from build123d import *

# Parameters (mm, degrees)
SKETCH1_R                      = 14
BOSS_EXTRUDE1_DEPTH            = 20
CIRPATTERN1_COUNT              = 3
CIRPATTERN1_ANGLE              = 90
M5X0_8_TAPPED_HOLE2_AT_2_COUNT = 2
M5X0_8_TAPPED_HOLE2_AT_2_PITCH = 24
CHAMFER1_SIZE                  = 0.5
FILLET1_R                      = 0.5


with BuildPart() as part:
    # Sketch1 → Boss-Extrude1 (new body, symmetric)
    with BuildSketch(Plane.XY):
        Polygon((-13.25, -19.5), (13.25, -19.5), (26, -6.75), (26, 20), (-26, 20), (-26, -6.75), align=None)
        Circle(SKETCH1_R, mode=Mode.SUBTRACT)
    extrude(amount=BOSS_EXTRUDE1_DEPTH, both=True)

    # Sketch4 → M5x0.8 Tapped Hole1 (revolve, cut)
    with BuildSketch(Plane(origin=(13.435028843, 13.435028843, -20), x_dir=(0, 1, 0), z_dir=(1, 0, 0))):
        Polygon((0, 0), (0, 16.9218073), (2.1, 15.66), (2.1, 0), align=None)
    m5x0_8_tapped_hole1 = revolve(axis=Axis((13.435028843, 13.435028843, -26.35), (0, 0, 1)), mode=Mode.SUBTRACT)

    # CirPattern1: M5x0.8 Tapped Hole1 ×3 about axis
    cirpattern1_axis = Axis((0, 0, 0), (0, 0, -1))
    for i in range(1, CIRPATTERN1_COUNT):
        add(m5x0_8_tapped_hole1.rotate(cirpattern1_axis, i * CIRPATTERN1_ANGLE / (CIRPATTERN1_COUNT - 1)), mode=Mode.SUBTRACT)

    # Mirror1: M5x0.8 Tapped Hole1 across plane
    add(m5x0_8_tapped_hole1.mirror(Plane(origin=(0, 0, 0), x_dir=(0, 0, 1), z_dir=(1, 0, 0))), mode=Mode.SUBTRACT)

    # Mirror1 copy 1 sketch → Mirror1 copy 1 (revolve, cut)
    with BuildSketch(Plane(origin=(-19, 0, -20), x_dir=(-0.707106781, 0.707106781, 0), z_dir=(-0.707106781, -0.707106781, 0))):
        Polygon((0, 0), (0, -16.9218073), (2.1, -15.66), (2.1, 0), align=None)
    revolve(axis=Axis((-19, 0, -26.35), (0, 0, -1)), mode=Mode.SUBTRACT)

    # Mirror1 copy 2 sketch → Mirror1 copy 2 (revolve, cut)
    with BuildSketch(Plane(origin=(-13.435028843, -13.435028843, -20), x_dir=(-1, 0, 0), z_dir=(0, -1, 0))):
        Polygon((0, 0), (0, -16.9218073), (2.1, -15.66), (2.1, 0), align=None)
    revolve(axis=Axis((-13.435028843, -13.435028843, -26.35), (0, 0, -1)), mode=Mode.SUBTRACT)

    # Sketch6 → M5x0.8 Tapped Hole2 (revolve, cut)
    with BuildSketch(Plane(origin=(-20, 20, -12), x_dir=(0, 0, 1), z_dir=(1, 0, 0))):
        Polygon((0, 0), (0, 16.7618073), (2.1, 15.5), (2.1, 0), align=None)
    m5x0_8_tapped_hole2 = revolve(axis=Axis((-20, 26.35, -12), (0, -1, 0)), mode=Mode.SUBTRACT)

    # M5x0.8 Tapped Hole2 at 2: M5x0.8 Tapped Hole2 ×2
    with Locations(*[(0, 0, i * M5X0_8_TAPPED_HOLE2_AT_2_PITCH) for i in range(1, M5X0_8_TAPPED_HOLE2_AT_2_COUNT)]):
        add(m5x0_8_tapped_hole2, mode=Mode.SUBTRACT)

    # Mirror2: M5x0.8 Tapped Hole2 across plane
    add(m5x0_8_tapped_hole2.mirror(Plane(origin=(0, 0, 0), x_dir=(0, 0, 1), z_dir=(1, 0, 0))), mode=Mode.SUBTRACT)

    # Mirror2 copy 1 sketch → Mirror2 copy 1 (revolve, cut)
    with BuildSketch(Plane(origin=(20, 20, 12), x_dir=(0, 0, 1), z_dir=(-1, 0, 0))):
        Polygon((0, 0), (0, -16.7618073), (2.1, -15.5), (2.1, 0), align=None)
    revolve(axis=Axis((20, 26.35, 12), (0, 1, 0)), mode=Mode.SUBTRACT)

    # Chamfer1
    chamfer1_edges = [part.edges().sort_by_distance(p)[0] for p in [
        (0, 20, 20),
        (-26, 6.625, 20),
        (-14, 0, -20),
        (-14, 0, 20),
        (-19.625, -13.125, 20),
        (0, -19.5, 20),
        (19.625, -13.125, 20),
        (0, -19.5, -20),
        (-19.625, -13.125, -20),
        (-26, 6.625, -20),
        (0, 20, -20),
        (26, 6.625, -20),
        (19.625, -13.125, -20),
        (26, 6.625, 20),
    ]]
    chamfer(chamfer1_edges, length=CHAMFER1_SIZE)

    # Fillet1
    fillet1_edges = [part.edges().sort_by_distance(p)[0] for p in [
        (26, 20, 0),
        (26, -6.75, 0),
        (13.25, -19.5, 0),
        (-13.25, -19.5, 0),
        (-26, -6.75, 0),
        (-26, 20, 0),
    ]]
    fillet(fillet1_edges, radius=FILLET1_R)


solid = part.part
Source: CAD feature listing. Evaluate the final solid. Frame: model axes, mm. A direction names the side the tool comes from. Round coordinates to 2 decimals unless told otherwise and drop trailing zeros. Order: outer loops, then holes, each group sorted by start corner. A loop starts at its lowest first (then second) coordinate and runs counter-clockwise, first axis right, second up. Notation, with made-up numbers: (-4, 79.5) -> (41, 79.5) arc R17 cw to (41, 112.5) -> close; hole circle Ø9 at (-28, 16.5). An arc over 180 degrees is marked (long way). Answer as CSV lines item,"result".
Item 1: Pull-direction query (X, two-part tool) for faces 1 (the face through (-19.86, 3.46, 12.34)), 2 (the face through (-19.71, -13.04, 0.27)), 3 (the face through (0, 20, 0)); classes: pulls with the +X half, pulls with the -X half, needs draft (parallel to the pull), parting line crosses it, or undercut.
A:
face 1,"undercut"
face 2,"pulls with the -X half"
face 3,"needs draft"
Item 2: Section B-B, the plane y = 10.5. Count the separate pieces of the cut face and the enclosed holes in it, plus the area to 3 significant figures.
A:
separate pieces,"2"
enclosed holes,"4"
area,"1,280 mm²"
Item 3: Line query: L1, parallel to Z at x = -20, y = 8; L2, parallel to Z at x = 20.5, y = 6; L3, parallel to X at y = 15, z = -17.5. Output: solid intervals per line, ascending.
A:
L1,"-20 to -14.1, -9.9 to 9.9, 14.1 to 20"
L2,"-20 to -14.04, -9.96 to 9.96, 14.04 to 20"
L3,"-26 to -14.84, -12.03 to 12.03, 14.84 to 26"
Item 4: Section A-A, the plane x = 0. Return loops of the section in (y, z), plus the area to 3 significant figures.
A:
outline,"(-19.5, -19.5) -> (-19, -20) -> (-14.5, -20) -> (-14, -19.5) -> (-14, 19.5) -> (-14.5, 20) -> (-19, 20) -> (-19.5, 19.5) -> close; (14, -19.5) -> (14.5, -20) -> (19.5, -20) -> (20, -19.5) -> (20, 19.5) -> (19.5, 20) -> (14.5, 20) -> (14, 19.5) -> close"
area,"459 mm²"
Item 5: Reachability of faces 4 (the face through (-21.003, -0.632, -12.28)), 5 (the face through (12.932, -5.362, -0.273)), 6 (the face through (22.082, 12.358, -12.273)) from +Z, -Z, +X, -X, +Y, -Y: full face, straight path, thin tool, end or side. Return the list, or none.
A:
face 4,"-Z"
face 5,"+Z, -Z"
face 6,"+Y"
Item 6: Pin query (flat end, axial travel): pin 1 Ø4 at (x, y) = (19, 0) entering from -Z; pin 2 Ø3.5 at (x, y) = (13.44, 13.44) entering from -Z; pin 3 Ø3.5 at (x, z) = (-20, -12) entering from -Y. Return the tip coordinate at first contact, or that it passes through.
A:
pin 1,"z = -4.28"
pin 2,"z = -4.13"
pin 3,"y = -14.5"
